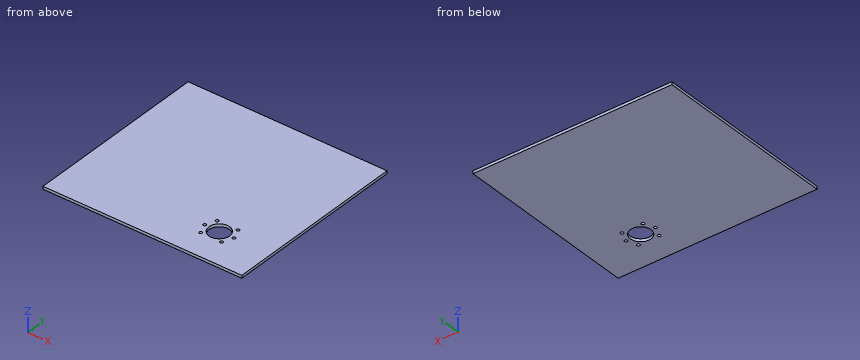
```python
from build123d import *

# Parameters (mm, degrees)
SKETCH_1_W          = 216
SKETCH_1_H          = 200
EXTRUDE_1_DEPTH     = 3
SKETCH_2_R          = 11.25
CUT_EXTRUDE_1_DEPTH = 148.217526131
HOLE_WIZARD_M4_1_D  = 3.3


with BuildPart() as part:
    # 草图1 → 凸台-拉伸1 (new body)
    with BuildSketch(Plane.XY):
        Rectangle(SKETCH_1_W, SKETCH_1_H)
    extrude(amount=EXTRUDE_1_DEPTH)

    # 草图2 → 切除-拉伸1 (cut, through all)
    with BuildSketch(Plane.XY.offset(3)):
        with Locations((52, -60)):
            Circle(SKETCH_2_R)
    extrude(amount=-CUT_EXTRUDE_1_DEPTH, mode=Mode.SUBTRACT)

    # M4 螺纹孔的螺纹孔钻头1 (through all)
    with Locations(Plane(origin=(36, -60, 3), x_dir=(1, 0, 0), z_dir=(0, 0, 1))):
        with Locations((0, 0), (4.686291501, 11.313708499), (4.686291501, -11.313708499), (27.313708499, 11.313708499), (32, 0), (27.313708499, -11.313708499)):
            Hole(HOLE_WIZARD_M4_1_D / 2)


solid = part.part
```
The model under review builds one solid part; all positions refer to its coordinate system, in mm. Round coordinates to 2 decimals unless told otherwise and drop trailing zeros. Loops run counter-clockwise (first coordinate to the right, second up) from the corner with the lowest first, then second, coordinate; pieces in that order, holes last. Notation, with made-up numbers: (-29.75, 30.5) - (-8.75, 30.5) arc R23 cw to (-8.75, 50.5) - close; hole circle Ø2 at (52, 62.5). An arc over 180 degrees is marked (long way). Write each question's results on one line, items separated by ' | '. Start each with the question number.
Q1. Wall thickness on line 1 along Y through (x, z) = (36, 1.05); line 2 along X through (y, z) = (-57.5, 2.45); line 3 along X through (y, z) = (-63.5, 1.8): over which ranges is each line inside the solid? List them lowest first. Write a range as [from, to].
Q2. Take a section at A-A on x = 52. Give the boundary of the cut face in (y, z), plus the area to 4 significant figures.
Q3. Take a section at B-B on y = -67. Give the boundary of the cut face in (x, z).
Q4. Insertion check: P1, Ø3, axis at x = 63.31, y = -48.69, coming from the -Z side. The pin has a flat end and moves straight along its axis. Give the tip position at first contact, or say it passes through.
Data:
1) line 1: y = [-100, -61.65], [-58.35, 100] | line 2: x = [-108, 41.03], [62.97, 108] | line 3: x = [-108, 41.31], [62.69, 108]
2) outline: (-100, 0) - (-71.25, 0) - (-71.25, 3) - (-100, 3) - close; (-48.75, 0) - (100, 0) - (100, 3) - (-48.75, 3) - close | area: 532.5 mm²
3) outline: (-108, 0) - (43.19, 0) - (43.19, 3) - (-108, 3) - close; (60.81, 0) - (108, 0) - (108, 3) - (60.81, 3) - close
4) P1: passes through
